```python
from build123d import *

# Parameters (mm, degrees)
F0_W     = 1.8008393743
F0_H     = 15.4953580059
F1_DEPTH = 40
F2_R     = 2


with BuildPart() as f1:
    # F0 (on Right) → F1 (new body)
    with BuildSketch(Plane.YZ):
        Polygon((0, 14), (0, 0), (140, 0), (140, 20), (0, 28), align=None)
        with Locations((27.1479118072, 11.1200559583)):
            Rectangle(F0_W, F0_H, mode=Mode.SUBTRACT)
        Polygon((37.0253970758, 12.135783628), (43.4894269202, 3.3723769554), (41.3697948883, 3.3723769554), (35.7230951554, 10.8877442876), (34.0986091661, 9.4463945059), (34.0986091661, 3.3723769554), (32.2977697919, 3.3723769554), (32.2977697919, 18.8677349612), (34.0986091661, 18.8677349612), (34.0986091661, 11.1827970664), (41.1256132782, 18.8677349612), (43.2554195439, 18.8677349612), align=None, mode=Mode.SUBTRACT)
        Polygon((50.3468604697, 12.135783628), (56.8108903141, 3.3723769554), (54.6912582823, 3.3723769554), (49.0445585493, 10.8877442876), (47.4200725601, 9.4463945059), (47.4200725601, 3.3723769554), (45.6192331858, 3.3723769554), (45.6192331858, 18.8677349612), (47.4200725601, 18.8677349612), (47.4200725601, 11.1827970664), (54.4470766722, 18.8677349612), (56.5768829378, 18.8677349612), align=None, mode=Mode.SUBTRACT)
        with BuildLine():
            Line((68.8402260215, 18.8677349612), (70.6410653957, 18.8677349612))
            Line((70.6410653957, 18.8677349612), (70.6410653957, 8.8427233032))
            add(Edge.make_bspline(
                [(70.6410653957, 8.8427233032), (70.6410653957, 6.1906397049), (69.0403192853, 4.6746788757)],
                knots=[0, 0, 0, 1, 1, 1], degree=2))
            add(Edge.make_bspline(
                [(69.0403192853, 4.6746788757), (67.4395731748, 3.1587180465), (64.6416588927, 3.1587180465)],
                knots=[0, 0, 0, 1, 1, 1], degree=2))
            add(Edge.make_bspline(
                [(64.6416588927, 3.1587180465), (61.8437446106, 3.1587180465), (60.3125224308, 4.6865488151)],
                knots=[0, 0, 0, 1, 1, 1], degree=2))
            add(Edge.make_bspline(
                [(60.3125224308, 4.6865488151), (58.781300251, 6.2143795837), (58.781300251, 8.8834202382)],
                knots=[0, 0, 0, 1, 1, 1], degree=2))
            Line((58.781300251, 8.8834202382), (58.781300251, 18.8677349612))
            Line((58.781300251, 18.8677349612), (60.5855310365, 18.8677349612))
            Line((60.5855310365, 18.8677349612), (60.5855310365, 8.757938022))
            add(Edge.make_bspline(
                [(60.5855310365, 8.757938022), (60.5855310365, 6.8180507864), (61.6453470525, 5.7785832379)],
                knots=[0, 0, 0, 1, 1, 1], degree=2))
            add(Edge.make_bspline(
                [(61.6453470525, 5.7785832379), (62.7051630684, 4.7391156895), (64.7603582865, 4.7391156895)],
                knots=[0, 0, 0, 1, 1, 1], degree=2))
            add(Edge.make_bspline(
                [(64.7603582865, 4.7391156895), (66.7205939896, 4.7391156895), (67.7804100055, 5.7836703548)],
                knots=[0, 0, 0, 1, 1, 1], degree=2))
            add(Edge.make_bspline(
                [(67.7804100055, 5.7836703548), (68.8402260215, 6.8282250201), (68.8402260215, 8.7782864895)],
                knots=[0, 0, 0, 1, 1, 1], degree=2))
            Line((68.8402260215, 8.7782864895), (68.8402260215, 18.8677349612))
        make_face(mode=Mode.SUBTRACT)
        with BuildLine():
            Line((86.8452283531, 18.8677349612), (86.8452283531, 3.3723769554))
            Line((86.8452283531, 3.3723769554), (84.7900331349, 3.3723769554))
            Line((84.7900331349, 3.3723769554), (76.3216792412, 16.3750476917))
            Line((76.3216792412, 16.3750476917), (76.2368939599, 16.3750476917))
            add(Edge.make_bspline(
                [(76.2368939599, 16.3750476917), (76.4064645225, 14.0858450973), (76.4064645225, 12.1798719742)],
                knots=[0, 0, 0, 1, 1, 1], degree=2))
            Line((76.4064645225, 12.1798719742), (76.4064645225, 3.3723769554))
            Line((76.4064645225, 3.3723769554), (74.7412815982, 3.3723769554))
            Line((74.7412815982, 3.3723769554), (74.7412815982, 18.8677349612))
            Line((74.7412815982, 18.8677349612), (76.7761283488, 18.8677349612))
            Line((76.7761283488, 18.8677349612), (85.2241337751, 5.9159353936))
            Line((85.2241337751, 5.9159353936), (85.3089190564, 5.9159353936))
            add(Edge.make_bspline(
                [(85.3089190564, 5.9159353936), (85.2885705888, 6.2008139387), (85.2139595413, 7.7540802917)],
                knots=[0, 0, 0, 1, 1, 1], degree=2))
            add(Edge.make_bspline(
                [(85.2139595413, 7.7540802917), (85.1393484938, 9.3073466446), (85.1596969613, 9.9754546611)],
                knots=[0, 0, 0, 1, 1, 1], degree=2))
            Line((85.1596969613, 9.9754546611), (85.1596969613, 18.8677349612))
            Line((85.1596969613, 18.8677349612), (86.8452283531, 18.8677349612))
        make_face(mode=Mode.SUBTRACT)
        Polygon((102.7102501853, 3.3723769554), (100.8449739972, 3.3723769554), (98.9152609954, 8.3000975031), (92.7055869948, 8.3000975031), (90.7996138717, 3.3723769554), (88.9750346187, 3.3723769554), (95.099923338, 18.932171775), (96.6158841672, 18.932171775), align=None, mode=Mode.SUBTRACT)
        with BuildLine():
            ThreePointArc((19.5, 14), (12, 6.5), (4.5, 14))
            ThreePointArc((4.5, 14), (12, 21.5), (19.5, 14))
        make_face(mode=Mode.SUBTRACT)
    extrude(amount=F1_DEPTH)

    # F2
    f2_edges = [f1.edges().sort_by_distance(p)[0] for p in [
        (20, 140, 20),
        (20, 0, 28),
        (20, 0, 0),
        (20, 140, 0),
    ]]
    fillet(f2_edges, radius=F2_R)


solid = f1.part
```
Design review of the part built by this model. Coordinates are the model's own, in mm. Coordinates: 2 decimals unless noted, no trailing zeros. Loops run counter-clockwise (first coordinate to the right, second up) from the corner with the lowest first, then second, coordinate; pieces in that order, holes last. Notation, with made-up numbers: (68.5, 58.25) - (114.5, 58.25) arc R3 cw to (114.5, 62.25) - close; hole circle Ø6 at (37.25, 4). An arc over 180 degrees is marked (long way). Use CSV: the item, a comma, the result in double quotes. Start each with the question number.
1) Consider section B-B on x = 31. Give the number of separate pieces and of enclosed holes in the cut face, then the cut area to 3 significant figures.
2) Consider section C-C on y = 52. Write out the cut boundary in (x, z), then the cut area to 3 significant figures.
3) Wall thickness on L1, parallel to Z at x = 20, y = 42; L2, parallel to Z at x = 9, y = 37.5; L3, parallel to Z at x = 16, y = 12: over which ranges is each line inside the solid? List them lowest first. Write a range as from..to.
4) For pin 1 Ø1.4 at (x, y) = (18, 27) entering from +Z; pin 2 Ø1.7 at (x, y) = (28.5, 55.5) entering from +Z; pin 3 Ø10 at (x, y) = (10, 79) entering from +Z, all flat-tipped, find the tip position at first contact; note any pin that passes through.
5) Consider section A-A on y = 12. Write out the cut boundary in (x, z), then the cut area to 3 significant figures.
6) The part is to be moulded in two halves that separate along Y. For faces 1 (the flat face through (19.72, 71.07, 23.94)), 2 (the flat face through (20, 28.048, 11)), 3 (the flat face through (20, 69, 0)), say which applies: +Y half, -Y half, draft (parallel to the pull), parting line (faces both ways), or undercut.
Geometry says:
1,separate pieces,"1"
1,enclosed holes,"7"
1,area,"2,800 mm^2"
2,outline,"(0, 0) - (40, 0) - (40, 6.95) - (0, 6.95) - close; (0, 9.89) - (40, 9.89) - (40, 13.92) - (0, 13.92) - close; (0, 16.19) - (40, 16.19) - (40, 25.03) - (0, 25.03) - close"
2,area,"793 mm^2"
3,L1,"0..3.37, 5.39..17.51, 18.87..25.6"
3,L2,"0..8.52, 11.49..12.65, 14.9..25.86"
3,L3,"0..6.5, 21.5..27.31"
4,pin 1,"z = 26.5"
4,pin 2,"z = 24.88"
4,pin 3,"z = 23.77"
5,outline,"(0, 0) - (40, 0) - (40, 6.5) - (0, 6.5) - close; (0, 21.5) - (40, 21.5) - (40, 27.31) - (0, 27.31) - close"
5,area,"493 mm^2"
6,face 1,"+Y half"
6,face 2,"undercut"
6,face 3,"draft"
